Here's the drawing with two shaded views (mm, measured from the low corner). I have some questions. A direction names the side the tool comes from. Round coordinates to 2 decimals unless told otherwise and drop trailing zeros.
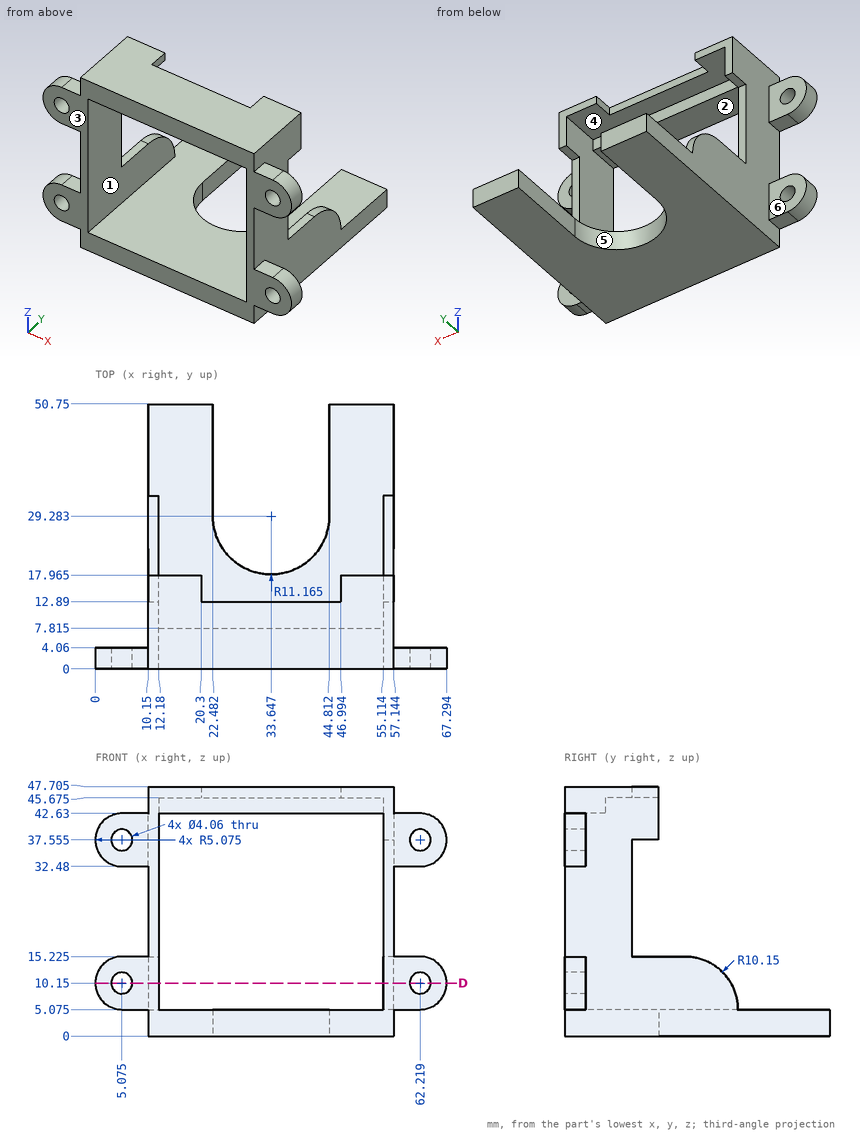
Item 1: For the marked faces 4, 5 and 6, which set-ups out of +Z, -Z, +X, -X, +Y, -Y let a thin tool reach every point of the face, with its end or its side?
Results list:
face 4: +Y
face 5: +Z, -Z, +Y
face 6: +Z, -Z, -X, +Y
Item 2: If I drill on line 1 along Z through (x, y) = (50.5, 5) (1 decimal); line 2 along Z through (x, y) = (50, 9.5) (1 decimal); line 3 along Z through (x, y) = (55.5, 36) (1 decimal), over which ranges is the centre line in solid material (lowest first)?
Results list:
line 1: z = 0 to 5.1, 42.6 to 47.7
line 2: z = 0 to 5.1, 45.7 to 47.7
line 3: z = 0 to 5.1
Item 3: If we section it at D-D, the plane z = 10.15: Count the separate pieces of the cut face and the enclosed holes in it, then the cut area to 3 significant figures.
Results list:
separate pieces: 4
enclosed holes: 0
area: 179 mm2
Item 4: Will these pins go through, and if not, where does the flat tip stop? pin 1 (1.2 mm diameter, centred on x = 7, y = 3, fed in from +Z); pin 2 (0.6 mm diameter, centred on x = 29.5, z = 46.5, fed in from +Y); pin 3 (5 mm diameter, centred on y = 11.5, z = 36.5, fed in from -X).
Results list:
pin 1: stops at z = 42.63
pin 2: stops at y = 12.89
pin 3: stops at x = 10.15
Item 5: We'd pull the mould along X, two halves only. Please class the marked faces 1, 2 and 3: released by +X, released by -X, zero draft, split by the parting line, or undercut.
Results list:
face 1: undercut
face 2: undercut
face 3: zero draft
